from build123d import *

# Parameters (mm, degrees)
SKETCH_1_R        = 30
EXTRUDE_1_DEPTH   = 10
SWEEP_1_PROFILE_R = 10
SKETCH_7_R        = 200
EXTRUDE_2_DEPTH   = 10


with BuildPart() as part:
    # Эскиз1 → Бобышка-Вытянуть1 (new body)
    with BuildSketch(Plane.XY):
        Circle(SKETCH_1_R)
    extrude(amount=EXTRUDE_1_DEPTH)

    # По траектории1: sweep along a curve in space
    with BuildLine() as sweep_1_path:
        Line((0, 0, 0), (0, 0, 300))
        Line((0, 0, 300), (0, -40, 300))
    # По траектории1 profile (on start of the path) → По траектории1 (sweep)
    with BuildSketch(Plane.XY):
        Circle(SWEEP_1_PROFILE_R)
    sweep(path=sweep_1_path.line, transition=Transition.RIGHT)

    # Эскиз7 → Бобышка-Вытянуть2 (add)
    with BuildSketch(Plane(origin=(0, -40, 0), x_dir=(-1, 0, 0), z_dir=(0, -1, 0))):
        with Locations(Location((0, -300, 0), (0, 0, 90))):
            Circle(SKETCH_7_R)
    extrude(amount=EXTRUDE_2_DEPTH)


solid = part.part
The listing builds one solid part. Answer for the finished solid, in the listing's coordinates (mm). Coordinates: 2 decimals unless noted, no trailing zeros. Write each loop counter-clockwise with the first axis right and the second up, starting at its lowest first coordinate (ties: lowest second). Pieces come first, ordered by that corner, then holes. Notation, with made-up numbers: M 11,-12.75 L 47,-12.75 A10 cw 47,3.25 Z; hole C 0,64 d4. An arc over 180 degrees is marked long. Use one line per item in the form item = value.
Item 1: Find section C-C, the plane x = 0. Give the vertices of the cut face in (y, z).
Model answer:
outline = M -50,100 L -40,100 L -40,290 L -10,290 L -10,10 L -30,10 L -30,0 L 30,0 L 30,10 L 10,10 L 10,310 L -40,310 L -40,500 L -50,500 Z
Item 2: Find section D-D, the plane z = 223. Give the vertices of the cut face in (x, y), plus the area to 3 significant figures.
Model answer:
outline = M -184.58,-50 L 184.58,-50 L 184.58,-40 L -184.58,-40 Z; C 0,0 d20
area = 4,010 mm2
Item 3: Find section A-A, the plane y = -24. Give the vertices of the cut face in (x, z), plus the area to 3 significant figures.
Model answer:
outline = M -18,0 L 18,0 L 18,10 L -18,10 Z; C 0,300 d20
area = 674 mm2
Item 4: Given P1, Ø3, axis at x = -17.5, y = 18, coming from the +Z side; P2, Ø5, axis at x = 40, z = 106, coming from the +Y side, each flat-ended and moving along its own axis, determine where each tip first touches the part or whether it passes through.
Model answer:
P1 = 10
P2 = -40
Item 5: The mould has two halves that part along Y. Classify faces 1 (the face through (5.38, 8.43, 162.1)), 2 (the face through (3, -50, 303)), 3 (the face through (-29.97, 1.32, 4.93)), 4 (the face through (0, 0, 0)): released by +Y, released by -Y, zero draft, split by the parting line, or undercut.
Model answer:
face_1 = undercut
face_2 = released by -Y
face_3 = split by the parting line
face_4 = zero draft
Item 6: Find section B-B, the plane z = 300. Give the vertices of the cut face in (x, y).
Model answer:
outline = M -200,-50 L 200,-50 L 200,-40 L 10,-40 L 10,0 A10 ccw -10,0 L -10,-40 L -200,-40 Z
Item 7: Find the intervals of material crossed by probe 1 along Y at (x, z) = (125.5, 195); probe 2 along Z at (x, y) = (25, -14); probe 3 along Y at (x, z) = (-8.5, 218), in increasing order.
Model answer:
probe_1 = -50 to -40
probe_2 = 0 to 10
probe_3 = -50 to -40, -5.27 to 5.27
